Geometry: final body of the model. Coordinates: model frame, mm. A direction names the side the tool comes from. Give positions to 0.01 mm unless a question says otherwise; leave off trailing zeros. Order: outer loops, then holes, each group sorted by start corner. A loop starts at its lowest first (then second) coordinate and runs counter-clockwise, first axis right, second up. Notation, with made-up numbers: (87, 40) -> (100, 40) arc R14 ccw to (100, 59) -> close; hole circle Ø4 at (73, 26.25). An arc over 180 degrees is marked (long way). Answer in a Markdown table with one row per item. Add a question column.
Q1. Pull-direction query (X, two-part tool) for faces 5 (the face through (3, -18, -90)), 6 (the face through (-0.506, -22.994, 14.739)), 7 (the face through (0, -8, 2.5)); classes: +X half, -X half, draft (parallel to the pull), parting line (faces both ways), or undercut.
Q2. Cut plane A-A on x = 0. Return the cut outline in (y, z).
Q3. Cut plane C-C on z = -54. Return the cut outline in (x, y).
Q4. Cut plane D-D on x = -7. Return the cut outline in (y, z).
Q5. Cut plane B-B on y = -11. Return the cut outline in (x, z), and give its area (3 significant figures).
Q6. Set-up query: faces 1 (the face through (2, -21, -75)), 2 (the face through (-21, 0, -8)), 3 (the face through (-0.451, -20.495, 51.554)), 4 (the face through (0, -8, 0)). Return all of +Z, -Z, +X, -X, +Y, -Y with unobstructed straight access to the full face (end or side cutting, diameter ignored); none if empty.
Q7. Line query: line 1 along Z through (x, y) = (8, -17.5); line 2 along X through (y, z) = (-7, -55); line 3 along Z through (x, y) = (-7, -13). Output: solid intervals per line, ascending. Write a range as from..to.
Q8. Contact query for flat-ended pins moving along their axis: P1, Ø12, axis at x = 8, z = 46.5, coming from the +Y side (3 decimals); P2, Ø1, axis at y = -13.5, z = 13.5, coming from the +X side; P3, Ø3, axis at y = -4.5, z = -6.5, coming from the -X side. Output: stop coordinate, or through.
from build123d import *

# Parameters (mm, degrees)
F3_DEPTH = 2.5
F5_DEPTH = 20
F7_DEPTH = 192.001


with BuildPart() as f1:
    # F0 (on Front) → F1 (revolve)
    with BuildSketch(Plane.XZ):
        Polygon((20.5, 2.5), (0, 2.5), (0, 0), (20.5, 0), (20.5, -70), (18, -70), (18, -90), (20.5, -90), (20.5, -75), (23, -75), (23, 0), (23, 102), (20.5, 102), align=None)
    revolve(axis=Axis((0, 0, 1.25), (0, 0, 1)))

    # F2 (on face) → F3 (cut, through all)
    with BuildSketch(Plane.XY.offset(2.5)):
        with BuildLine():
            Line((0, 12.5), (16.248077, 12.5))
            ThreePointArc((16.248077, 12.5), (9.055385, 18.391574), (0, 20.5))
            Line((0, 20.5), (0, 12.5))
        make_face()
    extrude(amount=-F3_DEPTH, mode=Mode.SUBTRACT)

    # F4 (on face) → F5 (join, through all)
    with BuildSketch(Plane(origin=(0, 0, -90), x_dir=(1, 0, 0), z_dir=(0, 0, -1))):
        with BuildLine():
            ThreePointArc((-17.706597, 3.236729), (-18, 0), (-17.706597, -3.236729))
            ThreePointArc((-17.706597, -3.236729), (-14.75, 0), (-17.706597, 3.236729))
        make_face()
        with BuildLine():
            ThreePointArc((17.706597, -3.236729), (18, 0), (17.706597, 3.236729))
            ThreePointArc((17.706597, 3.236729), (14.75, 0), (17.706597, -3.236729))
        make_face()
    extrude(amount=-F5_DEPTH)

    # F6 (on face) → F7 (cut, through all)
    with BuildSketch(Plane.XY.offset(102)):
        with BuildLine():
            Line((-23, 0), (23, 0))
            ThreePointArc((23, 0), (0, 23), (-23, 0))
        make_face()
    extrude(amount=-F7_DEPTH, mode=Mode.SUBTRACT)


solid = f1.part
Completed:
| question | item | result |
|---|---|---|
| 1 | face 5 | draft |
| 1 | face 6 | parting line |
| 1 | face 7 | undercut |
| 2 | outline | (-23, -75) -> (-20.5, -75) -> (-20.5, -90) -> (-18, -90) -> (-18, -70) -> (-20.5, -70) -> (-20.5, 0) -> (0, 0) -> (0, 2.5) -> (-20.5, 2.5) -> (-20.5, 102) -> (-23, 102) -> close |
| 3 | outline | (-23, 0) arc R23 ccw to (23, 0) -> (20.5, 0) arc R20.5 cw to (-20.5, 0) -> close |
| 4 | outline | (-21.91, -75) -> (-19.27, -75) -> (-19.27, -90) -> (-16.58, -90) -> (-16.58, -70) -> (-19.27, -70) -> (-19.27, 0) -> (0, 0) -> (0, 2.5) -> (-19.27, 2.5) -> (-19.27, 102) -> (-21.91, 102) -> close |
| 5 | outline | (-20.2, -75) -> (-17.3, -75) -> (-17.3, -90) -> (-14.25, -90) -> (-14.25, -70) -> (-17.3, -70) -> (-17.3, 0) -> (17.3, 0) -> (17.3, -70) -> (14.25, -70) -> (14.25, -90) -> (17.3, -90) -> (17.3, -75) -> (20.2, -75) -> (20.2, 102) -> (17.3, 102) -> (17.3, 2.5) -> (-17.3, 2.5) -> (-17.3, 102) -> (-20.2, 102) -> close |
| 5 | area | 1,240 mm² |
| 6 | face 1 | -Z, -Y |
| 6 | face 2 | +Z, -Z, +X, -X, +Y |
| 6 | face 3 | +Z, +Y |
| 6 | face 4 | +Y |
| 7 | line 1 | z = -90..-70, 0..2.5 |
| 7 | line 2 | x = -21.91..-19.27, 19.27..21.91 |
| 7 | line 3 | z = 0..2.5 |
| 8 | P1 | stops at y = -14.975 |
| 8 | P2 | stops at x = 18.97 |
| 8 | P3 | stops at x = -22.8 |
